```python
from build123d import *

# Parameters (mm, degrees)
F0_W     = 50.8
F0_H     = 50.8
F1_DEPTH = 50.8
F2_W     = 25.4
F2_H     = 25.4
F3_DEPTH = 12.7
F4_R     = 12.922989
F5_DEPTH = 12.7
F6_R     = 14.193725
F7_DEPTH = 50.8


with BuildPart() as f1:
    # F0 (on Front) → F1 (new body)
    with BuildSketch(Plane.XZ):
        with Locations((9.258268, -3.338678)):
            Rectangle(F0_W, F0_H)
    extrude(amount=F1_DEPTH)

    # F2 (on face) → F3 (join)
    with BuildSketch(Plane.XZ.offset(50.8)):
        with Locations((9.928127, -0.762303)):
            Rectangle(F2_W, F2_H)
    extrude(amount=F3_DEPTH)

    # F4 (on face) → F5 (join)
    with BuildSketch(Plane.YZ.offset(34.658268)):
        with Locations((-26.678886, -4.678389)):
            Circle(F4_R)
    extrude(amount=F5_DEPTH)

    # F6 (on face) → F7 (cut)
    with BuildSketch(Plane.XY.offset(22.061322)):
        with Locations((7.542709, -26.106022)):
            Circle(F6_R)
    extrude(amount=-F7_DEPTH, mode=Mode.SUBTRACT)


solid = f1.part
```
CAD build for the part. Positions are in the model's coordinates, mm. A direction names the side the tool comes from. Round coordinates to 2 decimals unless told otherwise and drop trailing zeros. Write each loop counter-clockwise with the first axis right and the second up, starting at its lowest first coordinate (ties: lowest second). Pieces come first, ordered by that corner, then holes. Notation, with made-up numbers: M 21,16 L 64,16 A4 cw 64,20 Z; hole C 14,-5 d6. An arc over 180 degrees is marked long. One line per question, with ' | ' between items.
1. Mould opens along Y. For faces 1 (the cylindrical face through (4.466, -39.962, -2.983)), 2 (the cylindrical face through (40.92, -14.35, -0.8)), 3 (the flat face through (22.628, -57, -1)) say: pulls with the +Y half, pulls with the -Y half, needs draft (parallel to the pull), parting line crosses it, or undercut.
Working result:
face 1: undercut | face 2: parting line crosses it | face 3: needs draft
2. Pin check, flat tips, straight feed: pin 1 Ø8 at (y, z) = (-41.5, 14) entering from +X; pin 2 Ø14 at (y, z) = (-59.5, -5.5) entering from +X; pin 3 Ø4 at (x, y) = (13.5, -59.5) entering from -Z; pin 4 Ø22.5 at (x, y) = (7.54, -26.11) entering from -Z. Stop position of each tip, or through.
Working result:
pin 1: x = 34.66 | pin 2: x = 22.63 | pin 3: z = -13.46 | pin 4: through
3. Probe L1, parallel to X at y = -3, z = -27; L2, parallel to Y at x = 31, z = 19; L3, parallel to Z at x = 19.5, y = -59.5. List the from-to ranges inside material, lowest first. Write a range as from..to.
Working result:
L1: -16.14..34.66 | L2: -50.8..0 | L3: -13.46..11.94
4. Cut at B-B on x = 19. Write the cut outline in (y, z), and give its area (3 significant figures).
Working result:
outline: M -63.5,-13.46 L -50.8,-13.46 L -50.8,-28.74 L -34.48,-28.74 L -34.48,22.06 L -50.8,22.06 L -50.8,11.94 L -63.5,11.94 Z; M -17.73,-28.74 L 0,-28.74 L 0,22.06 L -17.73,22.06 Z | area: 2,050 mm2
5. Cut at C-C on y = -25. Write the cut outline in (x, z).
Working result:
outline: M -16.14,-28.74 L -6.61,-28.74 L -6.61,22.06 L -16.14,22.06 Z; M 21.69,-28.74 L 34.66,-28.74 L 34.66,-17.49 L 47.36,-17.49 L 47.36,8.14 L 34.66,8.14 L 34.66,22.06 L 21.69,22.06 Z
6. Which spindle directions (+Z, -Z, +X, -X, +Y, -Y) get a long thin tool onto all of the face, cutting with end or side? Do faces 4 (the flat face through (10, -57, 11.938)), 5 (the flat face through (10, -57, -13.462)), 6 (the flat face through (34.658, -14, 2)). Say none if no direction does.
Working result:
face 4: +Z, +X, -X, -Y | face 5: -Z, +X, -X, -Y | face 6: +X
7. Cut at A-A on z = 0.5. Write the cut outline in (x, y).
Working result:
outline: M -16.14,-50.8 L -2.77,-50.8 L -2.77,-63.5 L 22.63,-63.5 L 22.63,-50.8 L 34.66,-50.8 L 34.66,-38.52 L 47.36,-38.52 L 47.36,-14.84 L 34.66,-14.84 L 34.66,0 L -16.14,0 Z; hole C 7.54,-26.11 d28.39
8. Cut at D-D on y = -47. Write the cut outline in (x, z), and give its area (3 significant figures).
Working result:
outline: M -16.14,-28.74 L 34.66,-28.74 L 34.66,22.06 L -16.14,22.06 Z | area: 2,580 mm2
